Read the model definition and answer for the solid it produces. Units are mm, in the model's axes. Face numbers are marked on the shaded views. A direction names the side the tool comes from. Round coordinates to 2 decimals unless told otherwise and drop trailing zeros. Order: outer loops, then holes, each group sorted by start corner. A loop starts at its lowest first (then second) coordinate and runs counter-clockwise, first axis right, second up. Notation, with made-up numbers: (-19.5, 42) -> (7.5, 42) arc R23 cw to (7.5, 51) -> close; hole circle Ø8 at (-10.5, -5.75). An arc over 180 degrees is marked (long way). Answer as a JSON object with one key per item and string values. Group by question number.
Item 1: Consider probe 1 along Y at (x, z) = (0, 4.05); probe 2 along Y at (x, z) = (0, 1.05); probe 3 along X at (y, z) = (0.5, 2.45). Determine where each line is inside the solid, lowest interval first. Write a range as from..to.
Item 2: Given P1, Ø1.5, axis at x = 0, y = 3.5, coming from the -Z side; P2, Ø1.2, axis at x = -2.5, y = 0, coming from the +Z side; P3, Ø3, axis at x = 1, y = 1, coming from the +Z side; P4, Ø3, axis at y = -4.5, z = 1, coming from the +X side, each flat-ended and moving along its own axis, determine where each tip first touches the part or whether it passes through.
Item 3: Section C-C, the plane z = 4.15 is taken. Write down the section's boundary in (x, y).
Item 4: For the marked faces 4 and 5, determine the directions among +Z, -Z, +X, -X, +Y, -Y from which every point of the face is accessible in a straight line to the end or side of a thin tool.
Item 5: The mould has two halves that part along X. Classify the marked faces 1, 2 and 3: pulls with the +X half, pulls with the -X half, needs draft (parallel to the pull), parting line crosses it, or undercut.
Item 6: Section A-A, the plane y = 0 is taken. Write down the section's boundary in (x, z).
from build123d import *

# Parameters (mm, degrees)
SKETCH1_R           = 7.5
BOSS_EXTRUDE1_DEPTH = 5
SKETCH2_R           = 5
CUT_EXTRUDE1_DEPTH  = 2.5
CHAMFER1_SIZE       = 2.5
SKETCH3_R           = 1
CUT_EXTRUDE2_DEPTH  = 2.5


with BuildPart() as part:
    # Sketch1 → Boss-Extrude1 (new body)
    with BuildSketch(Plane.XY):
        Circle(SKETCH1_R)
    extrude(amount=BOSS_EXTRUDE1_DEPTH)

    # Sketch2 → Cut-Extrude1 (cut)
    with BuildSketch(Plane.XY.offset(5)):
        Circle(SKETCH2_R)
    extrude(amount=-CUT_EXTRUDE1_DEPTH, mode=Mode.SUBTRACT)

    # Chamfer1
    chamfer1_edges = [part.edges().sort_by_distance(p)[0] for p in [
        (-7.5, 0, 0),
    ]]
    chamfer(chamfer1_edges, length=CHAMFER1_SIZE)

    # Sketch3 → Cut-Extrude2 (cut)
    with BuildSketch(Plane.XY.offset(2.5)):
        with Locations((0, 2.5)):
            Circle(SKETCH3_R)
        with Locations((2.5, 0)):
            Circle(SKETCH3_R)
        with Locations((0, -2.5)):
            Circle(SKETCH3_R)
        with Locations((-2.5, 0)):
            Circle(SKETCH3_R)
    extrude(amount=-CUT_EXTRUDE2_DEPTH, mode=Mode.SUBTRACT)


solid = part.part
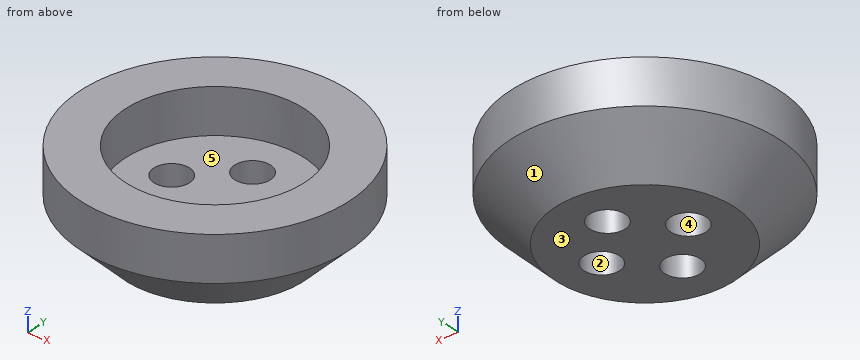
Values found:
{
 "1": {"probe 1": "-7.5..-5, 5..7.5", "probe 2": "-6.05..-3.5, -1.5..1.5, 3.5..6.05", "probe 3": "-7.43..-3.37, -1.63..1.63, 3.37..7.43"},
 "2": {"P1": "z = 0", "P2": "through", "P3": "z = 2.5", "P4": "x = 6.26"},
 "3": {"outline": "circle Ø15 at (0, 0); hole circle Ø10 at (0, 0)"},
 "4": {"face 4": "+Z, -Z", "face 5": "+Z"},
 "5": {"face 1": "parting line crosses it", "face 2": "undercut", "face 3": "needs draft"},
 "6": {"outline": "(-7.5, 2.5) -> (-5, 0) -> (-3.5, 0) -> (-3.5, 2.5) -> (-5, 2.5) -> (-5, 5) -> (-7.5, 5) -> close; (-1.5, 0) -> (1.5, 0) -> (1.5, 2.5) -> (-1.5, 2.5) -> close; (3.5, 0) -> (5, 0) -> (7.5, 2.5) -> (7.5, 5) -> (5, 5) -> (5, 2.5) -> (3.5, 2.5) -> close"}
}
